Could you check a few things on this model? Use its own coordinates, in mm. A direction names the side the tool comes from. Round coordinates to 2 decimals unless told otherwise and drop trailing zeros. Write each loop counter-clockwise with the first axis right and the second up, starting at its lowest first coordinate (ties: lowest second). Pieces come first, ordered by that corner, then holes. Notation, with made-up numbers: M 86.5,-24.75 L 108.5,-24.75 A26 ccw 108.5,0.25 Z; hole C 25,-30 d11. An arc over 180 degrees is marked long. One line per item, written item: value. Start each with the question number.
(1) Which directions (+Z, -Z, +X, -X, +Y, -Y) give clear straight access to the entire face, cutting with the end or side of a thin tool? Please do faces 1 (the face through (106, 10, -59)), 2 (the face through (39, 35, -80)), 3 (the face through (43, -3, -6)).
(2) I'm going to push flat-ended pins straight in: pin 1 Ø6 at (x, y) = (44.5, 14.5) entering from +Z; pin 2 Ø10 at (y, z) = (11, -50.5) entering from -X; pin 3 Ø1 at (x, z) = (45.5, -64) entering from +Y; pin 4 Ø3 at (x, z) = (83, -15) entering from +Y. Where does each tip first touch, or does it pass through?
(3) I want a section at A-A on x = 25.5. Please give me the cut outline in (y, z), and give its area (3 significant figures).
(4) If I drill on L1, parallel to X at y = 12.5, z = -40.5; L2, parallel to Z at x = 97, y = 36.5; L3, parallel to Y at x = 88.5, z = -18.5, over which ranges is the centre line in solid material (lowest first)?
(5) Thinking about a two-plate mould opening in Y: for faces 4 (the face through (0.601, 18.496, -38.268)), 5 (the face through (71.23, -2.13, -3.04)), 6 (the face through (110, 10, -49)), 7 (the face through (55, 0, -3)), which applies, released by +Y, released by -Y, zero draft, split by the parting line, or undercut?
Autodesk Inventor part; units mm, degrees
ref_plane "Work Plane1" through (106, 0, 0) normal (1, 0, 0) x (0, 0, -1)
ref_plane "YZ Plane" through (0, 0, 0) normal (1, 0, 0) x (0, 1, 0)
ref_plane "XY Plane" through (0, 0, 0) normal (0, 0, 1) x (1, 0, 0)
sketch "Sketch1" plane through (0, 0, 0) normal (1, 0, 0) x (0, 1, 0)
  line L0 (0, 0) -> (0, -80)
  line L1 (0, 0) -> (80, 0) construction
  line L2 (0, -80) -> (40, -80)
  line L3 (0, -80) -> (40, -80) construction
  line L4 (40, -80) -> (0, 0)
  dimension "d0" = 80
  dimension "d1" = 90
  dimension "d2" = 40
  dimension "d3" = 0
extrude "Extrusion1" add sketch "Sketch1" along normal blind 110
ref_plane "Work Plane1" through (106, 0, 0) normal (1, 0, 0) x (0, 0, -1)
sketch "Sketch2" plane through (106, 0, 0) normal (1, 0, 0) x (0, 0, -1)
  line L0 (0, 0) -> (80, 0)
  line L1 (80, 0) -> (80, 40)
  line L2 (80, 40) -> (0, 0)
  line L3 (0, 0) -> (80, 0)
  line L4 (80, 0) -> (80, 34)
  line L5 (80, 0) -> (80, 40)
  line L6 (80, 0) -> (114, 0) construction
  line L7 (80, 0) -> (6, 0)
  line L8 (80, 0) -> (154, 0) construction
  line L9 (6, 0) -> (80, 34)
  dimension "d7" = 34
  dimension "d8" = 90
  dimension "d9" = 74
  dimension "d10" = 180
extrude "Extrusion2" cut sketch "Sketch2" against normal blind 102 contours L9 L1 L0
sketch "Sketch3" plane through (0, 0, -80) normal (0, -1, 0) x (1, 0, 0)
  line L0 (0, 80) -> (0, 0) construction
  line L1 (0, 80) -> (37.5, 80) construction
  line L2 (0, 80) -> (37.5, 80) construction
  line L3 (106, 74) -> (106, 0) construction
  line L4 (106, 0) -> (110, 0) construction
  line L5 (110, 80) -> (110, 0) construction
  line L6 (0, 80) -> (110, 80) construction
  line L7 (0, 80) -> (0, 0) construction
  line L8 (0, 0) -> (4, 0) construction
  line L9 (4, 0) -> (4, 74) construction
  line L10 (4, 74) -> (106, 74) construction
  line L11 (110, 80) -> (110, 0) construction
  line L12 (110, 80) -> (72.5, 80) construction
  line L13 (0, 80) -> (110, 80) construction
  line L14 (110, 80) -> (147.5, 80) construction
  line L15 (37.5, 80) -> (47.5, 80)
  line L16 (47.5, 80) -> (47.5, 74)
  line L17 (47.5, 74) -> (37.5, 74)
  line L18 (37.5, 74) -> (37.5, 80)
  line L19 (72.5, 80) -> (62.5, 80)
  line L20 (62.5, 80) -> (62.5, 74)
  line L21 (62.5, 74) -> (72.5, 74)
  line L22 (72.5, 74) -> (72.5, 80)
  dimension "d13" = 37.5
  dimension "d14" = 0
  dimension "d17" = 37.5
  dimension "d18" = 180
  dimension "d21" = 10
  dimension "d22" = 6
  dimension "d23" = 10
  dimension "d24" = 6
extrude "Extrusion3" add sketch "Sketch3" along normal blind 4.33
draft "FaceDraft1" angle 30 pull direction (0, 1, 0) faces at (47.5, -1.4433, -2) fixed edges at (47.5, -4.33, -3)
draft "FaceDraft2" angle 30 pull direction (0, 1, 0) faces at (37.5, -1.4433, -4) fixed edges at (37.5, -4.33, -3)
draft "FaceDraft4" angle -30 pull direction (0, -1, 0) faces at (72.5, -1.4433, -4) fixed edges at (72.5, -4.33, -3)
fillet "Fillet2" radius 2 5 edges at (110, 20, -40) (110, 20, -80) (55, 40, -80) (0, 20, -80) (0, 20, -40)
draft "FaceDraft5" angle 30 pull direction (0, 1, 0) faces at (62.5, -1.4433, -2) fixed edges at (62.5, -4.33, -3)
properties part number "foot_cover_2_top"
Found:
1. face 1: -Z, -Y
1. face 2: -Z, +X, -X, +Y, -Y
1. face 3: -Z, +X, -X, -Y
2. pin 1: stops at z = -23
2. pin 2: stops at x = 0
2. pin 3: stops at y = 32.25
2. pin 4: stops at y = 8.25
3. outline: M 0,-6 L 34,-80 L 36.76,-80 A2 ccw 38.55,-77.11 L 0,0 Z
3. area: 340 mm²
4. L1: x = 0 to 4, 106 to 110
4. L2: z = -80 to -73
4. L3: y = 5.74 to 9.25
5. face 4: released by +Y
5. face 5: undercut
5. face 6: zero draft
5. face 7: undercut
